Build history of the part. All positions in model axes, mm. Face numbers are marked on the shaded views. Give positions to 0.01 mm unless a question says otherwise; leave off trailing zeros. Order: outer loops, then holes, each group sorted by start corner. A loop starts at its lowest first (then second) coordinate and runs counter-clockwise, first axis right, second up. Notation, with made-up numbers: (-30, -37.5) - (-24, -37.5) arc R25 ccw to (-24, -2.5) - close; hole circle Ø3 at (20.5, 64). An arc over 180 degrees is marked (long way). Use a Markdown table: item, result.
from build123d import *

# Parameters (mm, degrees)
F4_T     = -2.54
F6_DEPTH = 25.4
F6_TAPER = 4


with BuildPart() as f3:
    # F0 (on Top) → F3 section 0
    with BuildSketch(Plane.XY):
        with BuildLine():
            Line((37.4514907598, 59.8914325237), (0, 59.8914325237))
            Line((0, 59.8914325237), (-37.4514907598, 59.8914325237))
            ThreePointArc((-37.4514907598, 59.8914325237), (-41.9616667547, -3.1000974537), (0, -50.2964220941))
            ThreePointArc((0, -50.2964220941), (41.9616667547, -3.1000974537), (37.4514907598, 59.8914325237))
        make_face()
    # F2 (on offset) → F3 section 1
    with BuildSketch(Plane.XY.offset(38.1)):
        with BuildLine():
            Line((0, 60.5104640126), (-18.2614699006, 60.5104640126))
            ThreePointArc((-18.2614699006, 60.5104640126), (-14.7486334866, 17.3479007496), (0, -23.3684927225))
            ThreePointArc((0, -23.3684927225), (14.7486334866, 17.3479007496), (18.2614699006, 60.5104640126))
            Line((18.2614699006, 60.5104640126), (0, 60.5104640126))
        make_face()
    loft()

    # F4
    f4_openings = [f3.faces().sort_by_distance(p)[0] for p in [
        (0, 12.627016, 0),
    ]]
    offset(amount=F4_T, openings=f4_openings, kind=Kind.INTERSECTION)

    # F5 (on offset) → F6 (join)
    with BuildSketch(Plane.XY.offset(38.1)):
        Polygon((1.9884528592, 60.578674078), (0, 60.578674078), (-1.9884528592, 60.578674078), (-1.9884528592, 30.6487604976), (0, 30.6487604976), (1.9884528592, 30.6487604976), align=None)
    extrude(amount=F6_DEPTH, taper=F6_TAPER)


solid = f3.part
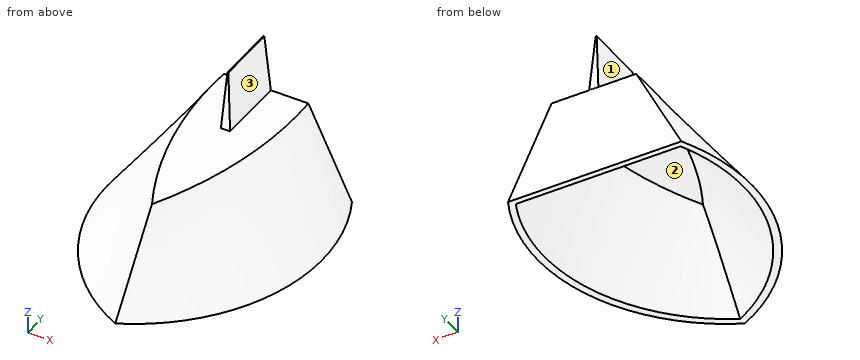
1) Slice it at B-B (z = 55). Write the cut outline in (x, y), and give its area (3 significant figures).
Computed:
| item | result |
|---|---|
| outline | (-0.81, 31.83) - (0.81, 31.83) - (0.81, 59.4) - (-0.81, 59.4) - close |
| area | 44.5 mm² |
2) Slice it at A-A (z = 45.5). Write the cut outline in (x, y), and give its area (3 significant figures).
Computed:
| item | result |
|---|---|
| outline | (-1.47, 31.17) - (1.47, 31.17) - (1.47, 60.06) - (-1.47, 60.06) - close |
| area | 85.0 mm² |
3) Two-plate mould, pull along X, no slides. Class the marked faces 1, 2 and 3: +X half, -X half, draft (parallel to the pull), parting line (faces both ways), or undercut.
Computed:
| item | result |
|---|---|
| face 1 | -X half |
| face 2 | undercut |
| face 3 | +X half |
4) Wall check: line 1 (X direction, y = -12.5, z = 6.5); line 2 (X direction, y = 20, z = 35); line 3 (X direction, y = 43, z = 36.5). Give the ranges that are in metal, low to high. Write a range as from..to.
Computed:
| item | result |
|---|---|
| line 1 | x = -31.9..-28.13, 28.13..31.9 |
| line 2 | x = -17.89..-14.54, 14.54..17.89 |
| line 3 | x = -19.39..19.39 |
5) Pin check, flat tips, straight feed: P1, Ø1, axis at x = 15, y = 44.5, coming from the -Z side; P2, Ø1, axis at x = 8, z = 9.5, coming from the +Y side; P3, Ø1, axis at x = -11.5, y = 23, coming from the +Z side. Stop position of each tip, or through.
Computed:
| item | result |
|---|---|
| P1 | stops at z = 35.56 |
| P2 | stops at y = 60.05 |
| P3 | stops at z = 38.1 |
